Study the drawing (mm; zero at the part's minimum x, y, z) and answer. Give positions to 0.01 mm unless a question says otherwise; leave off trailing zeros. Write each loop counter-clockwise with the first axis right and the second up, starting at its lowest first coordinate (ties: lowest second). Pieces come first, ordered by that corner, then holes. Notation, with made-up numbers: (40.5, 71.5) -> (53.5, 71.5) arc R21 ccw to (53.5, 100.5) -> close; hole circle Ø10 at (-23.75, 61.5). An arc over 180 degrees is marked (long way). Put each result on its own line as item: value. Start each with the question number.
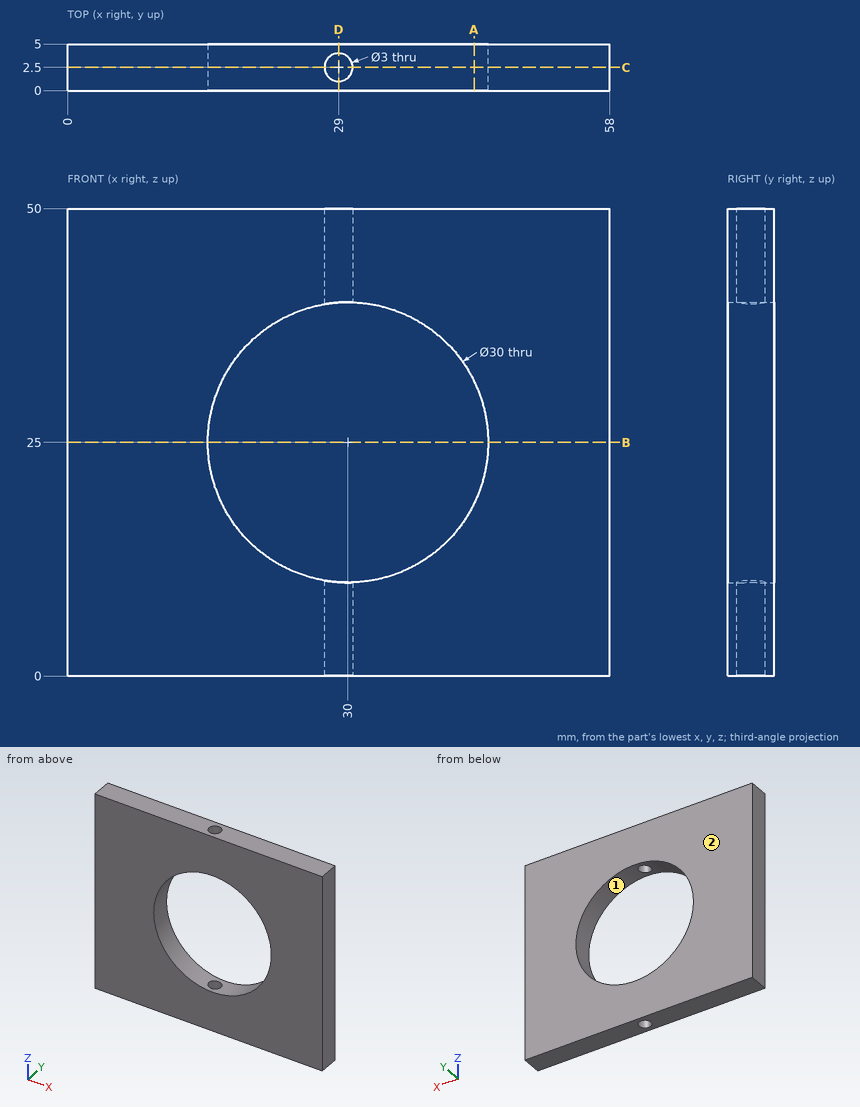
1) A cutting plane is placed at A-A on x = 43.5. Give the vertices of the cut face in (y, z).
2) This flat-tipped pin is pushed along its axis until it touches: pin 1 Ø8 at (x, z) = (27.5, 12) entering from -Y. Where does it stop, or does it pass through?
3) For a pull along X with two mould halves and no side action, classify the marked faces 1 and 2 as pulls with the +X half, pulls with the -X half, needs draft (parallel to the pull), parting line crosses it, or undercut.
4) Straight lines are drawn through the part: line 1 (Y direction, x = 29, z = 43.5); line 2 (X direction, y = 2.3, z = 4); line 3 (Z direction, x = 32, y = 4). For each, find the intervals that lie inside material, in ascending order. Write a range as [from, to].
5) A cutting plane is placed at D-D on x = 29. Give the vertices of the cut face in (y, z).
6) A cutting plane is placed at C-C on y = 2.5. Give the vertices of the cut face in (x, z), and give its area (3 significant figures).
7) A cutting plane is placed at B-B on z = 25. Give the vertices of the cut face in (x, y).
Results found:
1. outline: (0, 0) -> (5, 0) -> (5, 18.46) -> (0, 18.46) -> close; (0, 31.54) -> (5, 31.54) -> (5, 50) -> (0, 50) -> close
2. pin 1: stops at y = 0
3. face 1: undercut
3. face 2: needs draft
4. line 1: y = [0, 1], [4, 5]
4. line 2: x = [0, 27.51], [30.49, 58]
4. line 3: z = [0, 10.13], [39.87, 50]
5. outline: (0, 0) -> (1, 0) -> (1, 10.03) -> (0, 10.03) -> close; (0, 39.97) -> (1, 39.97) -> (1, 50) -> (0, 50) -> close; (4, 0) -> (5, 0) -> (5, 10.03) -> (4, 10.03) -> close; (4, 39.97) -> (5, 39.97) -> (5, 50) -> (4, 50) -> close
6. outline: (0, 0) -> (27.5, 0) -> (27.5, 10.21) arc R15 cw to (27.5, 39.79) -> (27.5, 50) -> (0, 50) -> close; (30.5, 0) -> (58, 0) -> (58, 50) -> (30.5, 50) -> (30.5, 39.99) arc R15 cw to (30.5, 10.01) -> close
6. area: 2,130 mm²
7. outline: (0, 0) -> (15, 0) -> (15, 5) -> (0, 5) -> close; (45, 0) -> (58, 0) -> (58, 5) -> (45, 5) -> close
